Part model, mm, in its own coordinate system. A direction names the side the tool comes from. Round coordinates to 2 decimals unless told otherwise and drop trailing zeros. Loops run counter-clockwise (first coordinate to the right, second up) from the corner with the lowest first, then second, coordinate; pieces in that order, holes last. Notation, with made-up numbers: (-35, -11) - (-3, -11) arc R17 cw to (-3, 9) - close; hole circle Ø8 at (61.5, 60.25). An arc over 180 degrees is marked (long way). Put each result on its own line as item: value.
Autodesk Inventor part; units mm, degrees
ref_plane "YZ Plane" through (0, 0, 0) normal (1, 0, 0) x (0, 1, 0)
ref_plane "XZ Plane" through (0, 0, 0) normal (0, 1, 0) x (-1, 0, 0)
ref_plane "XY Plane" through (0, 0, 0) normal (0, 0, 1) x (1, 0, 0)
sketch "Sketch1" plane through (0, 0, 0) normal (0, 1, 0) x (-1, 0, 0)
  line L0 (0, 0) -> (3, 0)
  line L1 (3, 0) -> (3, -20)
  line L2 (3, -20) -> (0, -20)
  line L3 (0, -20) -> (0, 0)
  line L4 (0, 0) -> (0, -8)
  circle A0 centre (0, -8) radius 1.55
  line L5 (3, 0) -> (6, 0)
  line L6 (6, 0) -> (6, -20)
  line L7 (6, -20) -> (3, -20)
  line L8 (0, 0) -> (3.15, 0)
  line L9 (3.15, 0) -> (3.15, 20)
  line L10 (3.15, 20) -> (0, 20)
  line L11 (0, 20) -> (0, 0)
  line L12 (0, 0) -> (0, 8)
  circle A1 centre (0, 8) radius 1.55
  line L13 (3.15, 20) -> (6, 20)
  line L14 (6, 20) -> (6, 0)
  circle A2 centre (0, -20) radius 1
  dimension "d0" = 3
  dimension "d1" = 20
  dimension "d2" = 3
  dimension "d3" = 8
  dimension "d4" = 3.1
  dimension "d5" = 3
  dimension "d6" = 3.15
  dimension "d7" = 20
  dimension "d8" = 8
  dimension "d9" = 3.1
  dimension "d11" = 2
revolve "Revolution1" add sketch "Sketch1" angle 360 about axis through (0, 0, 20) along (0, 0, -1) contours L5 L6 L7 L1 | L9 L13 L14 L5
extrude "Extrusion1" cut sketch "Sketch1" along normal mid plane 20 contours A0 L3 | L3 A0 | A1 L11 | L11 A1 | A2 L3 L2 | L2 L3 A2
properties part number "shaft_to_dc_coupler"
1. Band-saw the part on C-C (z = -8). List the corners of the cut face in (x, y).
A:
outline: (-1.55, -5.8) - (-1.55, -2.57) arc R3 cw to (-1.55, 2.57) - (-1.55, 5.8) arc R6 ccw to start; (1.55, -5.8) arc R6 ccw to (1.55, 5.8) - (1.55, 2.57) arc R3 cw to (1.55, -2.57) - close
2. Band-saw the part on B-B (y = 0). List the corners of the cut face in (x, z), plus the area to 3 significant figures.
A:
outline: (-6, -20) - (-3, -20) - (-3, 0) - (-3.15, 0) - (-3.15, 20) - (-6, 20) - close; (3, -20) - (6, -20) - (6, 20) - (3.15, 20) - (3.15, 0) - (3, 0) - close
area: 234 mm²
3. Pin check, flat tips, straight feed: P1, Ø4, axis at x = 3, z = 1, coming from the -Y side; P2, Ø5, axis at y = -4, z = 1.5, coming from the +X side; P3, Ø1.9, axis at x = 0, z = -8, coming from the -Y side; P4, Ø2, axis at x = 4, z = -12, coming from the -Y side. Stop position of each tip, or through.
A:
P1: stops at y = -5.92
P2: stops at x = 5.81
P3: passes through
P4: stops at y = -5.2
4. Band-saw the part on A-A (x = 0). List the corners of the cut face in (y, z).
A:
outline: (-6, -19) - (-3, -19) - (-3, -9.55) - (-6, -9.55) - close; (-6, -6.45) - (-3, -6.45) - (-3, 0) - (-3.15, 0) - (-3.15, 6.45) - (-6, 6.45) - close; (-6, 9.55) - (-3.15, 9.55) - (-3.15, 20) - (-6, 20) - close; (3, -19) - (6, -19) - (6, -9.55) - (3, -9.55) - close; (3, -6.45) - (6, -6.45) - (6, 6.45) - (3.15, 6.45) - (3.15, 0) - (3, 0) - close; (3.15, 9.55) - (6, 9.55) - (6, 20) - (3.15, 20) - close
5. Two-plate mould, pull along X, no slides. Class faces 3 (the flat face through (-3.5, 0.1, -20)), 4 (the cylindrical face through (-0.715, -4.348, 6.625)), 5 (the cylindrical face through (-2.769, -5.323, -0.28)): pulls with the +X half, pulls with the -X half, needs draft (parallel to the pull), parting line crosses it, or undercut.
A:
face 3: needs draft
face 4: undercut
face 5: parting line crosses it
6. Tool access for faces 1 (the cylindrical face through (0.41, -3.123, 10.14)), 2 (the flat face through (4, 0, -20)): list every direction of +Z, -Z, +X, -X, +Y, -Y with a clear straight run to the whole face (end or side of a thin tool).
A:
face 1: +Z
face 2: -Z, +X, -X, +Y, -Y
7. Probe line 1 along Z through (x, y) = (0, -5.15); line 2 along Y through (x, z) = (0, 10.5); line 3 along Y through (x, z) = (-0.75, -11.5). List the from-to ranges inside material, lowest first. Write a range as [from, to].
A:
line 1: z = [-19, -9.55], [-6.45, 6.45], [9.55, 20]
line 2: y = [-6, -3.15], [3.15, 6]
line 3: y = [-5.95, -2.9], [2.9, 5.95]
8. Band-saw the part on D-D (y = -4). List the corners of the cut face in (x, z).
A:
outline: (-4.47, -20) - (-1, -20) arc R1 cw to (1, -20) - (4.47, -20) - (4.47, 20) - (-4.47, 20) - close; hole circle Ø3.1 at (0, -8); hole circle Ø3.1 at (0, 8)
